The drawing under review shows one solid part. Ordinate dimensions are in mm from its lowest x, y, z. A direction names the side the tool comes from. Coordinates: 2 decimals unless noted, no trailing zeros. Loops run counter-clockwise (first coordinate to the right, second up) from the corner with the lowest first, then second, coordinate; pieces in that order, holes last. Notation, with made-up numbers: (36, -23.75) - (81, -23.75) arc R16 cw to (81, -10.75) - close; hole circle Ø11 at (56.25, 40). An arc over 180 degrees is marked (long way). Answer as a JSON object with one key per item and string values. Group by question number.
Item 1: To check wall thickness, follow line 1 (X direction, y = 4.25, z = 66.2); line 2 (Y direction, x = 36.5, z = 96.5); line 3 (Z direction, x = 7, y = 5.5). State the ranges of each line that lie inside material, in increasing order.
Item 2: Clearance check with flat-ended pins moving along their axes: pin 1 (2.5 mm diameter, centred on x = 86.05, z = 3.95, fed in from -Y); pin 2 (3.5 mm diameter, centred on y = 5, z = 107, fed in from -X); pin 3 (6 mm diameter, centred on x = 37, z = 92, fed in from +Y). State where each tip first meets the part, or that it passes through.
Item 3: Tool access review of the marked faces 1 and 2: name each direction out of +Z, -Z, +X, -X, +Y, -Y from which nothing blocks a thin tool from reaching the whole face with its end or side.
Item 4: We need section C-C (y = 5.5). Give the boundary of the cut face in (x, z), then the cut area to 3 significant figures.
Item 5: We need section B-B (x = 86.05). Give the boundary of the cut face in (y, z), then the cut area to 3 significant figures.
Item 6: We need section A-A (z = 3.95). Give the boundary of the cut face in (x, y).
Item 7: We need section D-D (x = 50). Give the boundary of the cut face in (y, z).
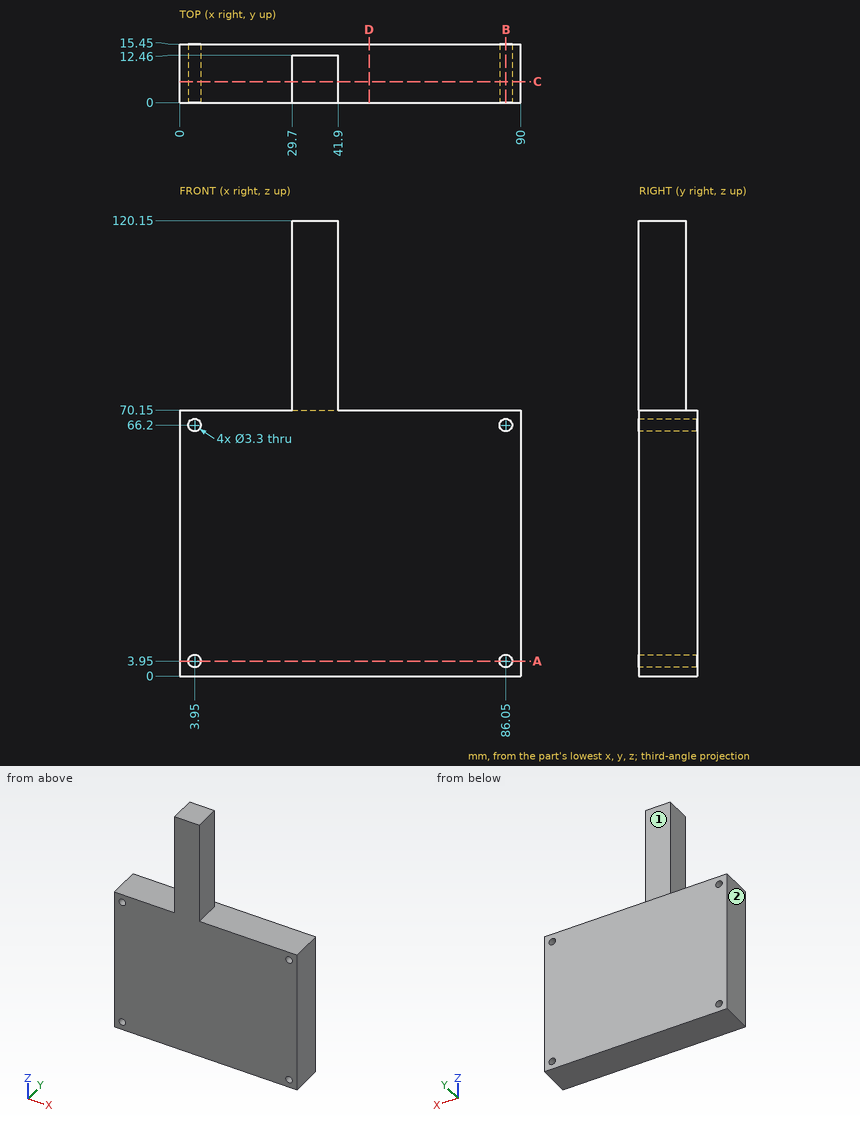
Check sheet entries:
{
 "1": {"line 1": "x = 0 to 2.3, 5.6 to 84.4, 87.7 to 90", "line 2": "y = 0 to 12.46", "line 3": "z = 0 to 70.15"},
 "2": {"pin 1": "passes through", "pin 2": "stops at x = 29.7", "pin 3": "stops at y = 12.46"},
 "3": {"face 1": "+Z, +X, -X, +Y", "face 2": "+Z, -Z, -X, +Y, -Y"},
 "4": {"outline": "(0, 0) - (90, 0) - (90, 70.15) - (41.9, 70.15) - (41.9, 120.15) - (29.7, 120.15) - (29.7, 70.15) - (0, 70.15) - close; hole circle Ø3.3 at (3.95, 3.95); hole circle Ø3.3 at (3.95, 66.2); hole circle Ø3.3 at (86.05, 3.95); hole circle Ø3.3 at (86.05, 66.2)", "area": "6,890 mm2"},
 "5": {"outline": "(0, 0) - (15.45, 0) - (15.45, 2.3) - (0, 2.3) - close; (0, 5.6) - (15.45, 5.6) - (15.45, 64.55) - (0, 64.55) - close; (0, 67.85) - (15.45, 67.85) - (15.45, 70.15) - (0, 70.15) - close", "area": "982 mm2"},
 "6": {"outline": "(0, 0) - (2.3, 0) - (2.3, 15.45) - (0, 15.45) - close; (5.6, 0) - (84.4, 0) - (84.4, 15.45) - (5.6, 15.45) - close; (87.7, 0) - (90, 0) - (90, 15.45) - (87.7, 15.45) - close"},
 "7": {"outline": "(0, 0) - (15.45, 0) - (15.45, 70.15) - (0, 70.15) - close"}
}
